Read the model definition and answer for the solid it produces. Units are mm, in the model's axes. Face numbers are marked on the shaded views. A direction names the side the tool comes from. Give positions to 0.01 mm unless a question says otherwise; leave off trailing zeros. Write each loop counter-clockwise with the first axis right and the second up, starting at its lowest first coordinate (ties: lowest second). Pieces come first, ordered by that corner, then holes.
Autodesk Inventor part; units mm, degrees
ref_plane "YZ Plane" through (0, 0, 0) normal (1, 0, 0) x (0, 1, 0)
ref_plane "XZ Plane" through (0, 0, 0) normal (0, 1, 0) x (-1, 0, 0)
ref_plane "XY Plane" through (0, 0, 0) normal (0, 0, 1) x (1, 0, 0)
sketch "Sketch1" plane through (0, 0, 0) normal (0, 0, 1) x (1, 0, 0)
  circle A0 centre (0, 0) radius 6
  circle A1 centre (0, 0) radius 7.5
  dimension "d0" = 12
  dimension "d1" = 15
extrude "Extrusion1" add sketch "Sketch1" along normal blind 49.288
sketch "Sketch2" plane through (0, 0, 0) normal (0, 0, -1) x (-1, 0, 0)
  circle A0 centre (0, 0) radius 4.1
  circle A1 centre (0, 0) radius 5
  dimension "d4" = 8.2
  dimension "d5" = 10
extrude "Extrusion2" add sketch "Sketch2" along normal blind 11.1125
sketch "Sketch3" plane through (0, 0, 0) normal (0, 0, -1) x (-1, 0, 0)
  circle A0 centre (0, 0) radius 4.1
  circle A1 centre (0, 0) radius 7.5
extrude "Extrusion3" add sketch "Sketch3" against normal blind 3.175
properties part number "OuterShaft" material "Steel, Alloy"
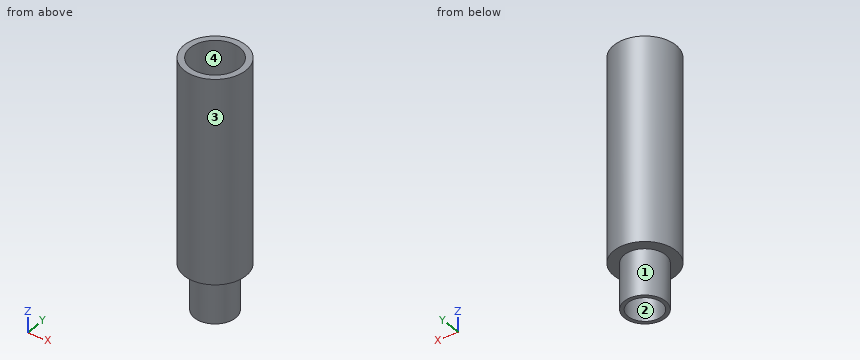
Item 1: Which of the six approach directions +Z, -Z, +X, -X, +Y, -Y give full straight-line access (tool end or side, diameter ignored) to the marked faces 3 and 4?
Result set:
face 3: +Z, -Z
face 4: +Z
Item 2: Section A-A (x = 0) is taken. Write down the section's boundary in (y, z) (1 decimal), and give its area (3 significant figures).
Result set:
outline: (-7.5, 0) - (-5, 0) - (-5, -11.1) - (-4.1, -11.1) - (-4.1, 3.2) - (-6, 3.2) - (-6, 49.3) - (-7.5, 49.3) - close; (4.1, -11.1) - (5, -11.1) - (5, 0) - (7.5, 0) - (7.5, 49.3) - (6, 49.3) - (6, 3.2) - (4.1, 3.2) - close
area: 180 mm2
Item 3: Find the intervals of material crossed by line 1 along Y through (x, z) = (0, 30); line 2 along Y through (x, z) = (0, -7.5); line 3 along Z through (x, y) = (-5, -4), in increasing order.
Result set:
line 1: y = -7.5 to -6, 6 to 7.5
line 2: y = -5 to -4.1, 4.1 to 5
line 3: z = 0 to 49.29
Item 4: Each of these flat-tipped pins is pushed along its axis until it touches: pin 1 Ø1 at (y, z) = (-2, -2.5) entering from +X; pin 2 Ø6 at (x, y) = (-1, 2) entering from +Z (3 decimals); pin 3 Ø3 at (x, z) = (-4, 26) entering from -Y. Where does it stop, or does it pass through?
Result set:
pin 1: stops at x = 4.77
pin 2: stops at z = 3.175
pin 3: stops at y = -7.07
Item 5: Determine the mould class of the marked faces 1 and 2 for opening direction X: pulls with the +X half, pulls with the -X half, needs draft (parallel to the pull), parting line crosses it, or undercut.
Result set:
face 1: parting line crosses it
face 2: undercut
Item 6: Section C-C (z = -1.5) is taken. Write down the section's boundary in (x, y), and give its area (3 significant figures).
Result set:
outline: circle Ø10 at (0, 0); hole circle Ø8.2 at (0, 0)
area: 25.7 mm2
